Autodesk Inventor part; units mm, degrees
ref_plane "YZ Plane" through (0, 0, 0) normal (1, 0, 0) x (0, 1, 0)
ref_plane "XZ Plane" through (0, 0, 0) normal (0, 1, 0) x (-1, 0, 0)
ref_plane "XY Plane" through (0, 0, 0) normal (0, 0, 1) x (1, 0, 0)
sketch "Sketch1" plane through (0, 0, 0) normal (0, 0, 1) x (1, 0, 0)
  line L0 (-35.56, 0) -> (35.56, 0) construction
  line L1 (0, -35.56) -> (0, 35.56) construction
  line L2 (-25.4, 25.4) -> (25.4, 25.4)
  line L3 (25.4, 25.4) -> (25.4, -25.4)
  line L4 (25.4, -25.4) -> (-25.4, -25.4)
  line L5 (-25.4, -25.4) -> (-25.4, 25.4)
  line L6 (-22.225, 22.225) -> (22.225, 22.225)
  line L7 (22.225, 22.225) -> (22.225, -22.225)
  line L8 (22.225, -22.225) -> (-22.225, -22.225)
  line L9 (-22.225, -22.225) -> (-22.225, 22.225)
  point P0 (0, 0)
  point P1 (-25.4, 0)
  point P2 (0, 25.4)
  point P3 (-22.225, 0)
  point P4 (0, 22.225)
  dimension "d0" = 50.8
  dimension "d1" = 3.175
extrude "Extrusion1" add sketch "Sketch1" along normal mid plane 215.9
sketch "Sketch2" plane through (25.4, -25.4, 107.95) normal (1, 0, 0) x (0, 0, -1)
  line L0 (268.3764, 25.4) -> (-44.7294, 25.4) construction
  line L1 (107.95, -10.16) -> (107.95, 60.96) construction
  line L2 (119.38, 7.62) -> (208.28, 7.62) construction
  line L3 (208.28, 7.62) -> (208.28, 43.18) construction
  line L4 (208.28, 43.18) -> (119.38, 43.18) construction
  line L5 (119.38, 43.18) -> (119.38, 7.62) construction
  circle A0 centre (119.38, 43.18) radius 2.667
  circle A1 centre (119.38, 7.62) radius 2.667
  circle A2 centre (163.83, 7.62) radius 2.667
  circle A3 centre (208.28, 7.62) radius 2.667
  circle A4 centre (208.28, 43.18) radius 2.667
  circle A5 centre (163.83, 43.18) radius 2.667
  line L6 (215.9, 50.8) -> (215.9, 0) construction
  point P0 (107.95, 25.4)
  point P1 (208.28, 25.4)
  dimension "d4" = 5.334
  dimension "d5" = 7.62
  dimension "d6" = 88.9
  dimension "d7" = 17.78
extrude "Extrusion2" cut sketch "Sketch2" against normal through all
sketch "Sketch4" plane through (-25.4, 25.4, 107.95) normal (0, 1, 0) x (1, 0, 0)
  line L0 (25.4, 259.08) -> (25.4, -43.18) construction
  line L1 (-10.16, 107.95) -> (60.96, 107.95) construction
  circle A0 centre (25.4, 19.05) radius 7.9375
  line L2 (50.8, 0) -> (0, 0) construction
  line L3 (38.1, 6.35) -> (12.7, 6.35) construction
  line L4 (12.7, 6.35) -> (12.7, 31.75) construction
  line L5 (12.7, 31.75) -> (38.1, 31.75) construction
  line L6 (38.1, 31.75) -> (38.1, 6.35) construction
  line L7 (38.1, 19.05) -> (12.7, 19.05) construction
  circle A1 centre (38.1, 6.35) radius 2.413 construction
  circle A2 centre (12.7, 6.35) radius 2.413 construction
  circle A3 centre (12.7, 31.75) radius 2.413 construction
  circle A4 centre (38.1, 31.75) radius 2.413 construction
  point P0 (25.4, 107.95)
  point P1 (25.4, 6.35)
  dimension "d13" = 15.875
  dimension "d14" = 19.05
  dimension "d17" = 4.826
  dimension "d18" = 25.4
extrude "Extrusion6" cut sketch "Sketch4" against normal up to next
properties part number "Arm 18 inch" material "Aluminum 6061"
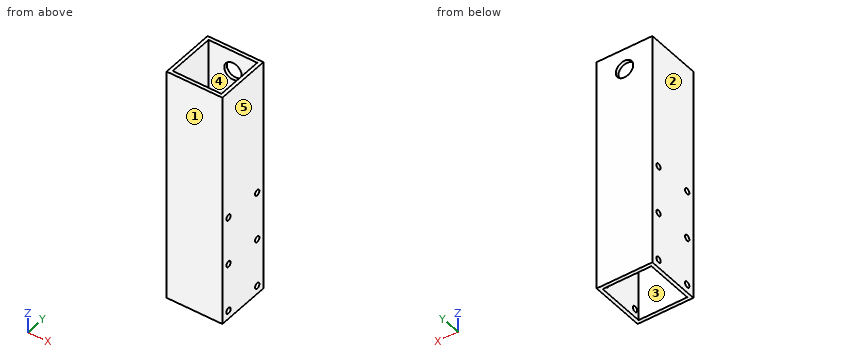
Work out the finished part from the listing and answer in its coordinate system (mm). Face numbers are marked on the shaded views. A direction names the side the tool comes from. Give positions to 0.01 mm unless a question says otherwise; leave off trailing zeros. Write each loop counter-clockwise with the first axis right and the second up, starting at its lowest first coordinate (ties: lowest second). Pieces come first, ordered by that corner, then holes.
Q1. A tool of negligible diameter and unlimited length cuts with its end or side. For the marked faces 4 and 5, from which of +Z, -Z, +X, -X, +Y, -Y can it reach the whole face along a straight path? Write none if from no direction.
Answer:
face 4: +Z, -Z
face 5: +Z, -Z, +X, +Y, -Y
Q2. Straight lines are drawn through the part: L1, parallel to Y at x = -23, z = -100; L2, parallel to X at y = -3, z = -96.5 (3 decimals). For each, find the intervals that lie inside material, in ascending order.
Answer:
L1: y = -25.4 to -20.43, -15.13 to 15.13, 20.43 to 25.4
L2: x = -25.4 to -22.225, 22.225 to 25.4
Q3. The part is cut by section D-D on z = 0. Give the vertices of the cut face in (x, y) (3 decimals).
Answer:
outline: (-25.4, -25.4) - (25.4, -25.4) - (25.4, 25.4) - (-25.4, 25.4) - close; hole (-22.225, -22.225) - (22.225, -22.225) - (22.225, 22.225) - (-22.225, 22.225) - close
Q4. The part is cut by section A-A on y = 17.78. State how many separate pieces and enclosed holes the cut face has, and give its area (3 significant figures).
Answer:
separate pieces: 8
enclosed holes: 0
area: 1,270 mm2
Q5. For a pull along Y with two mould halves and no side action, classify the marked faces 1, 2 and 3 as released by +Y, released by -Y, zero draft, split by the parting line, or undercut.
Answer:
face 1: released by -Y
face 2: zero draft
face 3: undercut
Q6. The part is cut by section B-B on y = -9. Give the vertices of the cut face in (x, z) (3 decimals).
Answer:
outline: (-25.4, -107.95) - (-22.225, -107.95) - (-22.225, 107.95) - (-25.4, 107.95) - close; (22.225, -107.95) - (25.4, -107.95) - (25.4, 107.95) - (22.225, 107.95) - close
